Model file for the job. Use its own axes, mm. A direction names the side the tool comes from. Give positions to 0.01 mm unless a question says otherwise; leave off trailing zeros. Write each loop counter-clockwise with the first axis right and the second up, starting at its lowest first coordinate (ties: lowest second). Pieces come first, ordered by that corner, then holes. Notation, with made-up numbers: (-9, -31.75) - (-3, -31.75) arc R17 cw to (-3, -20.75) - close; hole circle Ø10 at (-8.75, -30.75). An arc over 180 degrees is marked (long way). Use a Markdown table: item, result. Add a question column.
```python
from build123d import *

# Parameters (mm, degrees)
SKETCH2_W           = 101.6
SKETCH2_H           = 152.4
BOSS_EXTRUDE1_DEPTH = 3.175
SKETCH3_R           = 2.54
CUT_EXTRUDE1_DEPTH  = 4.175
SKETCH4_R           = 1.651
CUT_EXTRUDE2_DEPTH  = 4.175
SKETCH5_R           = 1.5875
CUT_EXTRUDE3_DEPTH  = 4.175
SKETCH6_W           = 6.35
SKETCH6_H           = 3.175
CUT_EXTRUDE4_DEPTH  = 4.175


with BuildPart() as part:
    # Sketch2 → Boss-Extrude1 (new body)
    with BuildSketch(Plane(origin=(0, 0, 0), x_dir=(1, 0, 0), z_dir=(0, 1, 0))):
        Rectangle(SKETCH2_W, SKETCH2_H)
    extrude(amount=BOSS_EXTRUDE1_DEPTH)

    # Sketch3 → Cut-Extrude1 (cut, through all)
    with BuildSketch(Plane(origin=(0, 3.175, 0), x_dir=(1, 0, 0), z_dir=(0, 1, 0))):
        with Locations((-38.1, -63.5)):
            Circle(SKETCH3_R)
        with Locations((-12.7, -63.5)):
            Circle(SKETCH3_R)
        with Locations((12.7, -63.5)):
            Circle(SKETCH3_R)
        with Locations((38.1, -63.5)):
            Circle(SKETCH3_R)
        with Locations((-38.1, -33.528)):
            Circle(SKETCH3_R)
        with Locations((-12.7, -33.528)):
            Circle(SKETCH3_R)
        with Locations((12.7, -33.528)):
            Circle(SKETCH3_R)
        with Locations((38.1, -33.528)):
            Circle(SKETCH3_R)
        with Locations((-12.7, 53.086)):
            Circle(SKETCH3_R)
        with Locations((-12.7, 23.114)):
            Circle(SKETCH3_R)
        with Locations((12.7, 23.114)):
            Circle(SKETCH3_R)
        with Locations((12.7, 53.086)):
            Circle(SKETCH3_R)
    extrude(amount=-CUT_EXTRUDE1_DEPTH, mode=Mode.SUBTRACT)

    # Sketch4 → Cut-Extrude2 (cut, through all)
    with BuildSketch(Plane(origin=(0, 3.175, 0), x_dir=(1, 0, 0), z_dir=(0, 1, 0))):
        with Locations((29.718, 13.589)):
            Circle(SKETCH4_R)
        with Locations((29.718, 21.971)):
            Circle(SKETCH4_R)
        with Locations((-29.718, 21.971)):
            Circle(SKETCH4_R)
        with Locations((-29.718, 13.589)):
            Circle(SKETCH4_R)
    extrude(amount=-CUT_EXTRUDE2_DEPTH, mode=Mode.SUBTRACT)

    # Sketch5 → Cut-Extrude3 (cut, through all)
    with BuildSketch(Plane(origin=(0, 3.175, 0), x_dir=(1, 0, 0), z_dir=(0, 1, 0))):
        with Locations((-24.13, 0)):
            Circle(SKETCH5_R)
        with Locations((24.13, 0)):
            Circle(SKETCH5_R)
        with Locations((-19.05, -50.8)):
            Circle(SKETCH5_R)
        with Locations((6.35, -50.8)):
            Circle(SKETCH5_R)
    extrude(amount=-CUT_EXTRUDE3_DEPTH, mode=Mode.SUBTRACT)

    # Sketch6 → Cut-Extrude4 (cut, through all)
    with BuildSketch(Plane(origin=(0, 3.175, 0), x_dir=(1, 0, 0), z_dir=(0, 1, 0))):
        with Locations((19.05, 68.2625)):
            Rectangle(SKETCH6_W, SKETCH6_H)
        with Locations((-19.05, 68.2625)):
            Rectangle(SKETCH6_W, SKETCH6_H)
    extrude(amount=-CUT_EXTRUDE4_DEPTH, mode=Mode.SUBTRACT)


solid = part.part
```
(1) Probe probe 1 along X at (y, z) = (2, -67.5) (3 decimals); probe 2 along X at (y, z) = (0.9, 0); probe 3 along Z at (x, y) = (-12.7, 2.15). List the from-to ranges inside material, lowest first. Write a range as [from, to].
(2) Band-saw the part on B-B (x = 24.13). Write the cut outline in (y, z) (1 decimal).
(3) Two-plate mould, pull along X, no slides. Class faces 1 (the flat face through (-1, 3.175, -1)), 2 (the cylindrical face through (10.684, 1.61, 65.046)): +X half, -X half, draft (parallel to the pull), parting line (faces both ways), or undercut.
(4) Band-saw the part on A-A (z = 63.5). Write the cut outline in (x, y) (3 decimals), then the cut area to 3 significant figures.
(5) Which spindle directions (+Z, -Z, +X, -X, +Y, -Y) get a long thin tool onto all of the face, cutting with end or side? Do faces 3 (the flat face through (-19, 2, -66.675)), 4 (the flat face through (-1, 2, 76.2)). Say none if no direction does.
(6) Band-saw the part on D-D (x = 12.7). Write the cut outline in (y, z) (3 decimals).
(7) Band-saw the part on C-C (x = 38.1). Write the cut outline in (y, z) (3 decimals), then the cut area to 3 significant figures.
Model answer:
| question | item | result |
|---|---|---|
| 1 | probe 1 | x = [-50.8, -22.225], [-15.875, 15.875], [22.225, 50.8] |
| 1 | probe 2 | x = [-50.8, -25.72], [-22.54, 22.54], [25.72, 50.8] |
| 1 | probe 3 | z = [-76.2, -55.63], [-50.55, -25.65], [-20.57, 30.99], [36.07, 60.96], [66.04, 76.2] |
| 2 | outline | (0, -76.2) - (3.2, -76.2) - (3.2, -1.6) - (0, -1.6) - close; (0, 1.6) - (3.2, 1.6) - (3.2, 76.2) - (0, 76.2) - close |
| 3 | face 1 | draft |
| 3 | face 2 | undercut |
| 4 | outline | (-50.8, 0) - (-40.64, 0) - (-40.64, 3.175) - (-50.8, 3.175) - close; (-35.56, 0) - (-15.24, 0) - (-15.24, 3.175) - (-35.56, 3.175) - close; (-10.16, 0) - (10.16, 0) - (10.16, 3.175) - (-10.16, 3.175) - close; (15.24, 0) - (35.56, 0) - (35.56, 3.175) - (15.24, 3.175) - close; (40.64, 0) - (50.8, 0) - (50.8, 3.175) - (40.64, 3.175) - close |
| 4 | area | 258 mm^2 |
| 5 | face 3 | +Y, -Y |
| 5 | face 4 | +Z, +X, -X, +Y, -Y |
| 6 | outline | (0, -76.2) - (3.175, -76.2) - (3.175, -55.626) - (0, -55.626) - close; (0, -50.546) - (3.175, -50.546) - (3.175, -25.654) - (0, -25.654) - close; (0, -20.574) - (3.175, -20.574) - (3.175, 30.988) - (0, 30.988) - close; (0, 36.068) - (3.175, 36.068) - (3.175, 60.96) - (0, 60.96) - close; (0, 66.04) - (3.175, 66.04) - (3.175, 76.2) - (0, 76.2) - close |
| 7 | outline | (0, -76.2) - (3.175, -76.2) - (3.175, 30.988) - (0, 30.988) - close; (0, 36.068) - (3.175, 36.068) - (3.175, 60.96) - (0, 60.96) - close; (0, 66.04) - (3.175, 66.04) - (3.175, 76.2) - (0, 76.2) - close |
| 7 | area | 452 mm^2 |
